from build123d import *

# Parameters (mm, degrees)
F1_DEPTH = 5
F2_SIZE2 = 3.124337
F2_SIZE  = 4.99999


# Not quite as in the source:
# - a fillet or chamfer is up to 0.001 mm smaller than in the source, because OpenCascade refuses the exact size


with BuildPart() as f1:
    # F0 (on Front) → F1 (new body)
    with BuildSketch(Plane.XZ):
        Polygon((-57.7801036188, 35.9519558773), (-52.0473758656, -43.8423787117), (25.6130563086, -63.0480360688), (67.8771152201, 4.8765494973), (16.3373079557, 66.061909406), align=None)
    extrude(amount=F1_DEPTH)

    # F2 (size 5 and 3.1243467595 in the source; OpenCascade refuses exactly that, so slightly less here)
    f2_edges = [f1.edges().sort_by_distance(p)[0] for p in [
        (-54.91374, -5, -3.945211),
        (-20.721398, -5, 51.006933),
        (42.107212, -5, 35.469229),
        (46.745086, -5, -29.085743),
        (-13.21716, -5, -53.445207),
    ]]
    chamfer(f2_edges, length=F2_SIZE, length2=F2_SIZE2)


solid = f1.part
Work out the finished part from the listing and answer in its coordinate system (mm). Coordinates: 2 decimals unless noted, no trailing zeros. Write each loop counter-clockwise with the first axis right and the second up, starting at its lowest first coordinate (ties: lowest second). Pieces come first, ordered by that corner, then holes. Notation, with made-up numbers: (21, 70.5) - (52, 70.5) arc R15 ccw to (52, 74.5) - close; hole circle Ø8 at (49.25, -20.5). An arc over 180 degrees is marked (long way). One line per question, with ' | ' between items.
1) Flat-ended cylindrical pins translate along their axes: P1, Ø3, axis at x = -25.5, y = -1, coming from the +Z side; P2, Ø2, axis at y = -3.5, z = 21.5, coming from the +X side; P3, Ø1, axis at y = -4, z = -34.5, coming from the -X side. Find the tip coordinate at first contact, or state that the pin passes through.
Checks:
P1: z = 49.52 | P2: x = 52.19 | P3: x = -50.53
2) Consider probe 1 along Z at (x, y) = (30.5, -2.65); probe 2 along X at (y, z) = (-0.85, 35); probe 3 along X at (y, z) = (-0.9, 43). Determine where each line is inside the solid, lowest interval first. Write a range as [from, to].
Checks:
probe 1: [-52.06, 46.68] | probe 2: [-57.18, 41.81] | probe 3: [-38.94, 35.03]
3) Find section B-B, the plane y = -0.8. Determine the outline of the cut face in (x, z), and give its area (3 significant figures).
Checks:
outline: (-57.26, 35.63) - (-51.57, -43.44) - (25.38, -62.48) - (67.26, 4.83) - (16.19, 65.46) - close | area: 10,800 mm2
